```python
from build123d import *

# Parameters (mm, degrees)
SKETCH_1_W          = 82
SKETCH_1_H          = 20
EXTRUDE_1_DEPTH     = 4
SKETCH_2_W          = 42
SKETCH_2_H          = 35
EXTRUDE_2_DEPTH     = 4
SKETCH_3_R          = 1.575
SKETCH_3_R_2        = 2.25
CUT_EXTRUDE_1_DEPTH = 87.580887036
FILLET_1_R          = 10


with BuildPart() as part:
    # 草图1 → 凸台-拉伸1 (new body)
    with BuildSketch(Plane.XY):
        with Locations((41, -10)):
            Rectangle(SKETCH_1_W, SKETCH_1_H)
    extrude(amount=EXTRUDE_1_DEPTH)

    # 草图2 → 凸台-拉伸2 (add)
    with BuildSketch(Plane.XY.offset(4)):
        with Locations((41, -10)):
            Rectangle(SKETCH_2_W, SKETCH_2_H)
    extrude(amount=-EXTRUDE_2_DEPTH)

    # 草图3 → 切除-拉伸1 (cut, through all)
    with BuildSketch(Plane.XY.offset(4)):
        with Locations((5, -5)):
            Circle(SKETCH_3_R)
        with Locations(Location((15, -5, 0), (0, 0, 180))):
            Circle(SKETCH_3_R)
        with Locations((15, -15)):
            Circle(SKETCH_3_R)
        with Locations(Location((5, -15, 0), (0, 0, 180))):
            Circle(SKETCH_3_R)
        with Locations((77, -15)):
            Circle(SKETCH_3_R)
        with Locations(Location((67, -15, 0), (0, 0, 180))):
            Circle(SKETCH_3_R)
        with Locations((67, -5)):
            Circle(SKETCH_3_R)
        with Locations(Location((77, -5, 0), (0, 0, 180))):
            Circle(SKETCH_3_R)
        with Locations((25.5, 2.5)):
            Circle(SKETCH_3_R_2)
        with Locations(Location((56.5, 2.5, 0), (0, 0, 180))):
            Circle(SKETCH_3_R_2)
        with Locations((56.5, -22.5)):
            Circle(SKETCH_3_R_2)
        with Locations(Location((25.5, -22.5, 0), (0, 0, 180))):
            Circle(SKETCH_3_R_2)
    extrude(amount=-CUT_EXTRUDE_1_DEPTH, mode=Mode.SUBTRACT)

    # 圆角1
    # the kernel refuses this fillet: 10 mm, written as the material it adds along each edge
    with BuildSketch(Plane(origin=(62, -20, 4), x_dir=(0, -1, 0), z_dir=(0, 0, -1)), Plane(origin=(62, 0, 0), x_dir=(0, 1, 0), z_dir=(0, 0, 1))) as fillet_1_piece_1:
        with BuildLine():
            CenterArc((10, -9.682458366), FILLET_1_R, 104.477512186, 75.522487814)
            Line((0, -9.682458366), (-0.2, -9.682458366))
            Line((-0.2, -9.682458366), (-0.2, 0))
            Line((-0.2, 0), (0, 0.2))
            ThreePointArc((0, 0.2), (3.75, 0.2), (7.45, 0.193649167))
            Line((7.45, 0.193649167), (7.5, 0))
        make_face()
    extrude(amount=4)
    with BuildSketch(Plane(origin=(20, -20, 0), x_dir=(-1, 0, 0), z_dir=(0, 0, 1)), Plane(origin=(20, 0, 4), x_dir=(-1, 0, 0), z_dir=(0, 0, -1))) as fillet_1_piece_2:
        with BuildLine():
            CenterArc((9.682458366, 10), FILLET_1_R, 194.477512186, 75.522487814)
            Line((0, 7.5), (-0.193649167, 7.45))
            ThreePointArc((-0.193649167, 7.45), (-0.2, 3.75), (-0.2, 0))
            Line((-0.2, 0), (0, -0.2))
            Line((0, -0.2), (9.682458366, -0.2))
            Line((9.682458366, -0.2), (9.682458366, 0))
        make_face()
    extrude(amount=4)


solid = part.part
```
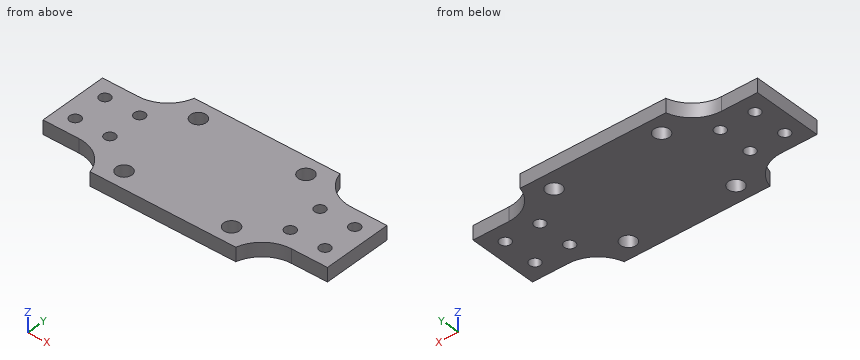
Input: part model. Units: mm. Frame: model coordinates. Coordinates: 2 decimals unless noted, no trailing zeros. Write each loop counter-clockwise with the first axis right and the second up, starting at its lowest first coordinate (ties: lowest second). Pieces come first, ordered by that corner, then holes.
1) Section C-C on z = 1.15. State how many separate pieces and enclosed holes the cut face has, and give its area (3 significant figures).
2) Section A-A on y = -5. Output: boundary loops of the cut face in (x, z) (3 decimals), and give its area (3 significant figures).
3) Section D-D on y = -22.5. Output: boundary loops of the cut face in (x, z).
4) Material intervals for line 1 along Y through (x, z) = (56.5, 1.65); line 2 along Y through (x, z) = (77, 1.3) (3 decimals); line 3 along X through (y, z) = (-23.5, 3.45), sorted ascending.
5) Pin query (flat end, axial travel): pin 1 Ø1.2 at (x, z) = (75.5, 2.5) entering from -Y; pin 2 Ø3.5 at (x, y) = (56.5, 2.5) entering from +Z; pin 3 Ø2 at (x, z) = (63.5, 2.5) entering from -Y. Return the tip coordinate at first contact, or that it passes through.
6) Section B-B on x = 56.5. Output: boundary loops of the cut face in (y, z), and give its area (3 significant figures).
Check result:
1. separate pieces: 1
1. enclosed holes: 12
1. area: 2,220 mm2
2. outline: (0, 0) - (3.425, 0) - (3.425, 4) - (0, 4) - close; (6.575, 0) - (13.425, 0) - (13.425, 4) - (6.575, 4) - close; (16.575, 0) - (65.425, 0) - (65.425, 4) - (16.575, 4) - close; (68.575, 0) - (75.425, 0) - (75.425, 4) - (68.575, 4) - close; (78.575, 0) - (82, 0) - (82, 4) - (78.575, 4) - close
2. area: 278 mm2
3. outline: (16.93, 0) - (23.25, 0) - (23.25, 4) - (16.93, 4) - close; (27.75, 0) - (54.25, 0) - (54.25, 4) - (27.75, 4) - close; (58.75, 0) - (65.07, 0) - (65.07, 4) - (58.75, 4) - close
4. line 1: y = -27.5 to -24.75, -20.25 to 0.25, 4.75 to 7.5
4. line 2: y = -20 to -16.575, -13.425 to -6.575, -3.425 to 0
4. line 3: x = 17.92 to 23.48, 27.52 to 54.48, 58.52 to 64.08
5. pin 1: stops at y = -20
5. pin 2: passes through
5. pin 3: stops at y = -26.04
6. outline: (-27.5, 0) - (-24.75, 0) - (-24.75, 4) - (-27.5, 4) - close; (-20.25, 0) - (0.25, 0) - (0.25, 4) - (-20.25, 4) - close; (4.75, 0) - (7.5, 0) - (7.5, 4) - (4.75, 4) - close
6. area: 104 mm2
